Check sheet for the drawn part. Datum: minimum x, y, z corner. Units: mm. Coordinates: 2 decimals unless noted, no trailing zeros. Loops run counter-clockwise (first coordinate to the right, second up) from the corner with the lowest first, then second, coordinate; pieces in that order, holes last.
Q1. Go/stop test with flat-tipped pins: P1, Ø6, axis at y = 6.5, z = 7.5, coming from the +X side; P2, Ø1, axis at y = 9, z = 11.5, coming from the +X side; P3, Ø5, axis at x = 17, y = 2, coming from the +Z side; P4, Ø6, axis at x = 22, z = 8.5, coming from the -Y side. Record where each tip stops, or that it passes through.
Q2. Sectioned sample at D-D (x = 4). Enter the section's corners in (y, z).
Q3. Sectioned sample at A-A (z = 6). Enter the section's corners in (x, y).
Q4. Mould release check, pull along X, two halves, no side actions. Record for the marked faces 1, 2, 3 and 4: +X half, -X half, draft (parallel to the pull), parting line (faces both ways), or undercut.
Q5. Material ranges on probe 1 along X at (y, z) = (3.5, 9); probe 2 along X at (y, z) = (5.75, 5.75) (1 decimal); probe 3 along Z at (x, y) = (19, 3.75) (1 decimal), recorded low to high.
Q6. Sectioned sample at C-C (z = 9). Enter the section's corners in (x, y).
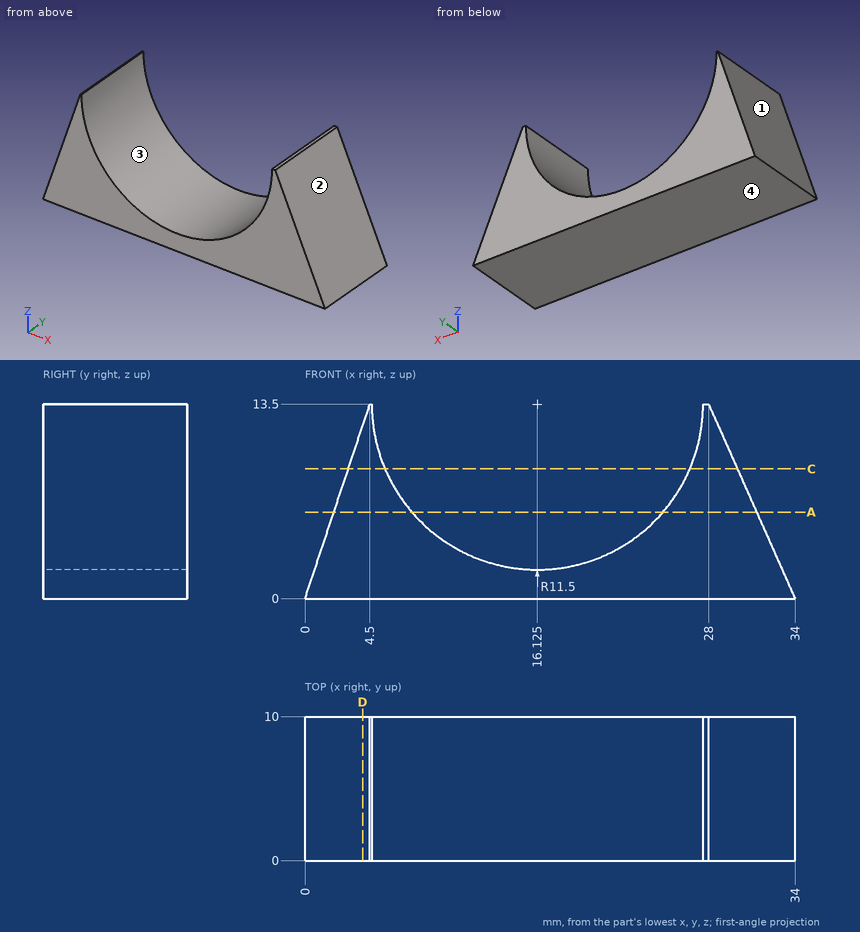
Geometry check:
1. P1: stops at x = 32
1. P2: stops at x = 29.11
1. P3: stops at z = 2.51
1. P4: passes through
2. outline: (0, 0) - (10, 0) - (10, 12) - (0, 12) - close
3. outline: (2, 0) - (7.41, 0) - (7.41, 10) - (2, 10) - close; (24.84, 0) - (31.33, 0) - (31.33, 10) - (24.84, 10) - close
4. face 1: -X half
4. face 2: +X half
4. face 3: undercut
4. face 4: draft
5. probe 1: x = 3 to 5.54, 26.71 to 30
5. probe 2: x = 1.9 to 7.6, 24.6 to 31.4
5. probe 3: z = 0 to 2.4
6. outline: (3, 0) - (5.54, 0) - (5.54, 10) - (3, 10) - close; (26.71, 0) - (30, 0) - (30, 10) - (26.71, 10) - close
